from build123d import *

# Parameters (mm, degrees)
SKETCH1_R           = 102.5
BOSS_EXTRUDE1_DEPTH = 7
SKETCH3_R           = 23.5
CUT_EXTRUDE1_DEPTH  = 146.125807491
SKETCH4_R           = 4
CUT_EXTRUDE2_DEPTH  = 5
CIRPATTERN1_COUNT   = 10
SKETCH5_R           = 102.5
BOSS_EXTRUDE2_DEPTH = 49
SKETCH6_R           = 3
CUT_EXTRUDE5_DEPTH  = 156.397876433


with BuildPart() as part:
    # Sketch1 → Boss-Extrude1 (new body)
    with BuildSketch(Plane.XY):
        Circle(SKETCH1_R)
    extrude(amount=BOSS_EXTRUDE1_DEPTH)

    # Sketch3 → Cut-Extrude1 (cut, through all)
    with BuildSketch(Plane.XY.offset(7)):
        Circle(SKETCH3_R)
    extrude(amount=-CUT_EXTRUDE1_DEPTH, mode=Mode.SUBTRACT)

    # Sketch4 → Cut-Extrude2 (cut)
    with BuildSketch(Plane.XY.offset(7)):
        with Locations((80, 0)):
            Circle(SKETCH4_R)
    cut_extrude2 = extrude(amount=-CUT_EXTRUDE2_DEPTH, mode=Mode.SUBTRACT)

    # CirPattern1: Cut-Extrude2 ×10 about axis
    cirpattern1_axis = Axis((0, 0, 0), (0, 0, 1))
    for i in range(1, CIRPATTERN1_COUNT):
        add(cut_extrude2.rotate(cirpattern1_axis, i * 360 / CIRPATTERN1_COUNT), mode=Mode.SUBTRACT)

    # Sketch5 → Boss-Extrude2 (add)
    with BuildSketch(Plane.XY.offset(7)):
        Circle(SKETCH5_R)
        with BuildLine():
            ThreePointArc((-13.256058456, 84.118628025), (-29.047597471, 89.399312532), (-38.719312427, 75.84511528))
            ThreePointArc((-38.719312427, 75.84511528), (-39.898528404, 70.960347818), (-43.304755731, 67.265876424))
            ThreePointArc((-43.304755731, 67.265876424), (-47.022820183, 64.72135955), (-50.59174464, 61.971569081))
            ThreePointArc((-50.59174464, 61.971569081), (-55.157977863, 59.873708832), (-60.168065566, 60.261683952))
            ThreePointArc((-60.168065566, 60.261683952), (-76.047597471, 55.251813715), (-75.905221984, 38.601346378))
            ThreePointArc((-75.905221984, 38.601346378), (-73.988033475, 33.956360727), (-74.572173468, 28.965340396))
            ThreePointArc((-74.572173468, 28.965340396), (-76.084521304, 24.72135955), (-77.355555556, 20.398971167))
            ThreePointArc((-77.355555556, 20.398971167), (-79.816624518, 16.017802027), (-84.097916667, 13.386824829))
            ThreePointArc((-84.097916667, 13.386824829), (-94, 0), (-84.097916667, -13.386824829))
            ThreePointArc((-84.097916667, -13.386824829), (-79.816624518, -16.017802027), (-77.355555556, -20.398971167))
            ThreePointArc((-77.355555556, -20.398971167), (-76.084521304, -24.72135955), (-74.572173468, -28.965340396))
            ThreePointArc((-74.572173468, -28.965340396), (-73.988033475, -33.956360727), (-75.905221984, -38.601346378))
            ThreePointArc((-75.905221984, -38.601346378), (-76.047597471, -55.251813715), (-60.168065566, -60.261683952))
            ThreePointArc((-60.168065566, -60.261683952), (-55.157977863, -59.873708832), (-50.59174464, -61.971569081))
            ThreePointArc((-50.59174464, -61.971569081), (-47.022820183, -64.72135955), (-43.304755731, -67.265876424))
            ThreePointArc((-43.304755731, -67.265876424), (-39.898528404, -70.960347818), (-38.719312427, -75.84511528))
            ThreePointArc((-38.719312427, -75.84511528), (-29.047597471, -89.399312532), (-13.256058456, -84.118628025))
            ThreePointArc((-13.256058456, -84.118628025), (-9.430858415, -80.859893896), (-4.503606821, -79.873133941))
            ThreePointArc((-4.503606821, -79.873133941), (0, -80), (4.503606821, -79.873133941))
            ThreePointArc((4.503606821, -79.873133941), (9.430858415, -80.859893896), (13.256058456, -84.118628025))
            ThreePointArc((13.256058456, -84.118628025), (29.047597471, -89.399312532), (38.719312427, -75.84511528))
            ThreePointArc((38.719312427, -75.84511528), (39.898528404, -70.960347818), (43.304755731, -67.265876424))
            ThreePointArc((43.304755731, -67.265876424), (47.022820183, -64.72135955), (50.59174464, -61.971569081))
            ThreePointArc((50.59174464, -61.971569081), (55.157977863, -59.873708832), (60.168065566, -60.261683952))
            ThreePointArc((60.168065566, -60.261683952), (76.047597471, -55.251813715), (75.905221984, -38.601346378))
            ThreePointArc((75.905221984, -38.601346378), (73.988033475, -33.956360727), (74.572173468, -28.965340396))
            ThreePointArc((74.572173468, -28.965340396), (76.084521304, -24.72135955), (77.355555556, -20.398971167))
            ThreePointArc((77.355555556, -20.398971167), (79.816624518, -16.017802027), (84.097916667, -13.386824829))
            ThreePointArc((84.097916667, -13.386824829), (94, 0), (84.097916667, 13.386824829))
            ThreePointArc((84.097916667, 13.386824829), (79.816624518, 16.017802027), (77.355555556, 20.398971167))
            ThreePointArc((77.355555556, 20.398971167), (76.084521304, 24.72135955), (74.572173468, 28.965340396))
            ThreePointArc((74.572173468, 28.965340396), (73.988033475, 33.956360727), (75.905221984, 38.601346378))
            ThreePointArc((75.905221984, 38.601346378), (76.047597471, 55.251813715), (60.168065566, 60.261683952))
            ThreePointArc((60.168065566, 60.261683952), (55.157977863, 59.873708832), (50.59174464, 61.971569081))
            ThreePointArc((50.59174464, 61.971569081), (47.022820183, 64.72135955), (43.304755731, 67.265876424))
            ThreePointArc((43.304755731, 67.265876424), (39.898528404, 70.960347818), (38.719312427, 75.84511528))
            ThreePointArc((38.719312427, 75.84511528), (29.047597471, 89.399312532), (13.256058456, 84.118628025))
            ThreePointArc((13.256058456, 84.118628025), (9.430858415, 80.859893896), (4.503606821, 79.873133941))
            ThreePointArc((4.503606821, 79.873133941), (0, 80), (-4.503606821, 79.873133941))
            ThreePointArc((-4.503606821, 79.873133941), (-9.430858415, 80.859893896), (-13.256058456, 84.118628025))
        make_face(mode=Mode.SUBTRACT)
    extrude(amount=BOSS_EXTRUDE2_DEPTH)

    # Sketch6 → Cut-Extrude5 (cut, through all)
    with BuildSketch(Plane.XY.offset(56)):
        with Locations((0, 90)):
            Circle(SKETCH6_R)
        with Locations((52.900672706, 72.811529494)):
            Circle(SKETCH6_R)
        with Locations((85.595086467, 27.811529494)):
            Circle(SKETCH6_R)
        with Locations((85.595086467, -27.811529494)):
            Circle(SKETCH6_R)
        with Locations((52.900672706, -72.811529494)):
            Circle(SKETCH6_R)
        with Locations((0, -90)):
            Circle(SKETCH6_R)
        with Locations((-52.900672706, -72.811529494)):
            Circle(SKETCH6_R)
        with Locations((-85.595086467, -27.811529494)):
            Circle(SKETCH6_R)
        with Locations((-85.595086467, 27.811529494)):
            Circle(SKETCH6_R)
        with Locations((-52.900672706, 72.811529494)):
            Circle(SKETCH6_R)
    extrude(amount=-CUT_EXTRUDE5_DEPTH, mode=Mode.SUBTRACT)


solid = part.part
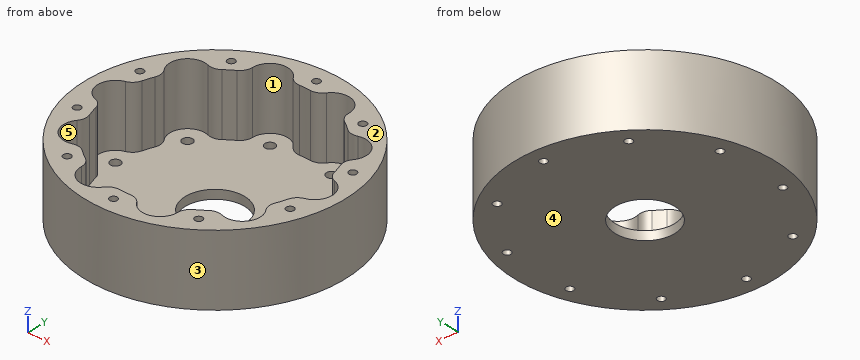
Read the model definition and answer for the solid it produces. Units are mm, in the model's axes. Face numbers are marked on the shaded views. A direction names the side the tool comes from. Give positions to 0.01 mm unless a question says otherwise; leave off trailing zeros. Loops run counter-clockwise (first coordinate to the right, second up) from the corner with the lowest first, then second, coordinate; pieces in that order, holes last. Notation, with made-up numbers: (-3.75, 7.25) - (46.25, 7.25) arc R26 ccw to (46.25, 32.25) - close; hole circle Ø4 at (63.5, 57.5). An arc over 180 degrees is marked (long way). Answer as CSV lines item,"result". Start each with the question number.
1) Find section B-B (x = 0). Write down the section's boundary in (y, z).
2) Straight lines are drawn through the part: L1, parallel to Y at x = 0, z = 3; L2, parallel to X at y = 81.5, z = 18.5; L3, parallel to X at y = -76, z = 51.5. For each, find the intervals that lie inside material, in ascending order. Write a range as from..to.
3) Find section C-C (z = 45.5). State how many separate pieces and enclosed holes the cut face has, then the cut area to 3 significant figures.
4) Each of these flat-tipped pins is pushed along its axis until it touches: pin 1 Ø9 at (x, y) = (-26, -76.5) entering from +Z; pin 2 Ø5 at (x, y) = (64.72, -47.02) entering from +Z; pin 3 Ø2 at (x, z) = (60.5, 13) entering from -Y. Where does it stop, or does it pass through?
5) Determine the mould class of the marked faces 1, 2 and 3 for opening direction X: released by +X, released by -X, zero draft, split by the parting line, or undercut.
6) Which of the six approach directions +Z, -Z, +X, -X, +Y, -Y give full straight-line access (tool end or side, diameter ignored) to the marked faces 4 and 5?
7) Find section A-A (y = 0). Write down the section's boundary in (x, z), then the cut area to 3 significant figures.
Findings below:
1,outline,"(-102.5, 0) - (-93, 0) - (-93, 56) - (-102.5, 56) - close; (-87, 0) - (-23.5, 0) - (-23.5, 7) - (-80, 7) - (-80, 56) - (-87, 56) - close; (23.5, 0) - (87, 0) - (87, 56) - (80, 56) - (80, 7) - (23.5, 7) - close; (93, 0) - (102.5, 0) - (102.5, 56) - (93, 56) - close"
2,L1,"-102.5..-93, -87..-23.5, 23.5..87, 93..102.5"
2,L2,"-62.16..-37.63, -10.56..10.56, 37.63..62.16"
2,L3,"-68.78..-38.72, 38.72..68.78"
3,separate pieces,"1"
3,enclosed holes,"11"
3,area,"9,280 mm^2"
4,pin 1,"z = 7"
4,pin 2,"z = 2"
4,pin 3,"y = -83.46"
5,face 1,"undercut"
5,face 2,"zero draft"
5,face 3,"split by the parting line"
6,face 4,"-Z, +X, -X, +Y, -Y"
6,face 5,"+Z"
7,outline,"(-102.5, 0) - (-23.5, 0) - (-23.5, 7) - (-76, 7) - (-76, 2) - (-84, 2) - (-84, 7) - (-94, 7) - (-94, 56) - (-102.5, 56) - close; (23.5, 0) - (102.5, 0) - (102.5, 56) - (94, 56) - (94, 7) - (84, 7) - (84, 2) - (76, 2) - (76, 7) - (23.5, 7) - close"
7,area,"1,860 mm^2"
